Input: part model. Units: mm. Frame: model coordinates. A direction names the side the tool comes from. Give positions to 0.01 mm unless a question says otherwise; leave off trailing zeros. Order: outer loops, then holes, each group sorted by start corner. A loop starts at its lowest first (then second) coordinate and runs counter-clockwise, first axis right, second up. Notation, with made-up numbers: (11.25, 11.25) -> (24.25, 11.25) arc R20 ccw to (24.25, 24.25) -> close; hole circle Ø10 at (2.5, 62.5). An arc over 180 degrees is marked (long way). Use a Markdown table: item, result. Add a question column.
from build123d import *

# Parameters (mm, degrees)
F0_R     = 5
F1_DEPTH = 15
F2_W     = 4
F2_H     = 4
F3_DEPTH = 10
F4_R     = 2
F5_SIZE  = 2


with BuildPart() as f1:
    # F0 (on Top) → F1 (new body)
    with BuildSketch(Plane.XY):
        Circle(F0_R)
    extrude(amount=F1_DEPTH)

    # F2 (on face) → F3 (cut)
    with BuildSketch(Plane.XY.offset(15)):
        Rectangle(F2_W, F2_H)
    extrude(amount=-F3_DEPTH, mode=Mode.SUBTRACT)

    # F4
    f4_edges = [f1.edges().sort_by_distance(p)[0] for p in [
        (-5, 0, 15),
    ]]
    fillet(f4_edges, radius=F4_R)

    # F5
    f5_edges = [f1.edges().sort_by_distance(p)[0] for p in [
        (-5, 0, 0),
    ]]
    chamfer(f5_edges, length=F5_SIZE)

    # F6: F1 across face


with BuildPart() as f1_1:
    add(f1.part)
    add(f1.part.mirror(Plane.XY.offset(15)))


solid = f1_1.part
Q1. Ray query, line 1 (Z direction, x = 1.5, y = -1); line 2 (Y direction, x = 0.25, z = 5.25); line 3 (Y direction, x = 0.75, z = 22.5). Return the intervals inside material, ascending.
Q2. Section query B-B (z = 10). Return loops of the section in (x, y), plus the area to 3 significant figures.
Q3. Draft query along Y for faces 3 (the cylindrical face through (-1.08, -4.88, 7.42)), 4 (the flat face through (0, 0, 30)), 5 (the flat face through (0, 0, 25)). Return one class per face: +Y half, -Y half, draft (parallel to the pull), parting line (faces both ways), or undercut.
Q4. First-contact query: pin 1 (1.5 mm diameter, centred on y = 3.5, z = 15.5, fed in from +X); pin 2 (1 mm diameter, centred on x = 1, z = 8, fed in from -Y); pin 3 (1.5 mm diameter, centred on x = 3, z = 17, fed in from -Y). Flat tips, straight axial feed; report the tip coordinate or a pass-through.
Q5. Section query A-A (y = 0). Return loops of the section in (x, z).
Q6. Access query for faces 1 (the flat face through (-2, 0, 15)), 2 (the flat face through (0, 0, 0)). Directions: +Z, -Z, +X, -X, +Y, -Y. A direction counts if a zero-diameter tool reaches every point of the face in a straight line with its end or side. Return the directions, or none.
Q7. Section query D-D (z = 26). Return loops of the section in (x, y), plus the area to 3 significant figures.
Solution:
| question | item | result |
|---|---|---|
| 1 | line 1 | z = 0 to 5, 25 to 30 |
| 1 | line 2 | y = -4.99 to -2, 2 to 4.99 |
| 1 | line 3 | y = -4.94 to -2, 2 to 4.94 |
| 2 | outline | circle Ø10 at (0, 0); hole (-2, -2) -> (2, -2) -> (2, 2) -> (-2, 2) -> close |
| 2 | area | 62.5 mm² |
| 3 | face 3 | parting line |
| 3 | face 4 | draft |
| 3 | face 5 | undercut |
| 4 | pin 1 | stops at x = 3.71 |
| 4 | pin 2 | stops at y = -4.97 |
| 4 | pin 3 | stops at y = -4.47 |
| 5 | outline | (-5, 2) -> (-3, 0) -> (3, 0) -> (5, 2) -> (5, 13) arc R2 ccw to (3, 15) arc R2 ccw to (5, 17) -> (5, 28) -> (3, 30) -> (-3, 30) -> (-5, 28) -> (-5, 17) arc R2 ccw to (-3, 15) arc R2 ccw to (-5, 13) -> close; hole (-2, 5) -> (2, 5) -> (2, 25) -> (-2, 25) -> close |
| 6 | face 1 | none |
| 6 | face 2 | -Z, +X, -X, +Y, -Y |
| 7 | outline | circle Ø10 at (0, 0) |
| 7 | area | 78.5 mm² |
